Print and shaded views of the part. All mm, measured from the part's lowest x, y and z. A direction names the side the tool comes from. Round coordinates to 2 decimals unless told otherwise and drop trailing zeros. Loops run counter-clockwise (first coordinate to the right, second up) from the corner with the lowest first, then second, coordinate; pieces in that order, holes last. Notation, with made-up numbers: (57, -30) - (89, -30) arc R25 cw to (89, -13) - close; hole circle Ø9 at (0, 12). An arc over 180 degrees is marked (long way). Use one line per item in the form item = value. Start each with the question number.
Q1. Saw through at C-C (z = 3.5). Give the cut face in (x, y) (1 decimal).
Q2. Saw through at B-B (x = 5.5). Give the cut face in (y, z).
Q3. Mould opens along X. For the marked faces 1, 2 and 3 say: released by +X, released by -X, zero draft, split by the parting line, or undercut.
Q4. Pin check, flat tips, straight feed: pin 1 (1 mm diameter, centred on y = 13.5, z = 5.5, fed in from +X); pin 2 (10 mm diameter, centred on x = 10, y = 10.5, fed in from +Z); pin 3 (1 mm diameter, centred on x = 2.5, z = 1.5, fed in from -Y); pin 4 (1.5 mm diameter, centred on x = 13, z = 7, fed in from -Y). Stop position of each tip, or through.
Q5. Saw through at A-A (y = 10). Give the cut face in (x, z).
Q6. 3-axis set-ups, long thin cutter, end or side, ignore diameter. For the marked faces 4 and 5: which of +Z, -Z, +X, -X, +Y, -Y reach the whole face in a straight line?
Q7. Drill centre lines: line 1 (Y direction, x = 10.5, z = 3.5); line 2 (Y direction, x = 4, z = 4) (1 decimal); line 3 (Y direction, x = 7.75, z = 7). Where is each one in solid material? Low to high.
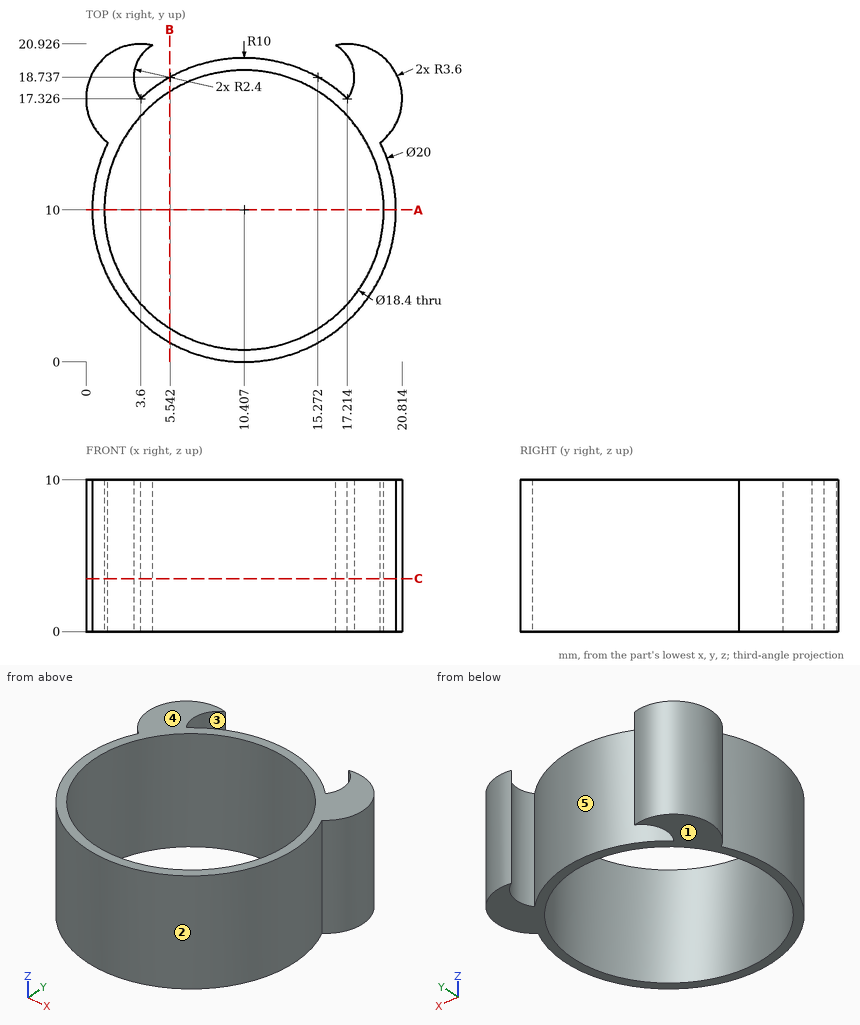
Report:
q1.outline = (1.4, 14.4) arc R10 ccw (long way) to (19.4, 14.4) arc R3.6 ccw to (16.4, 20.8) arc R2.4 cw to (17.2, 17.3) arc R10 ccw to (3.6, 17.3) arc R2.4 cw to (4.4, 20.8) arc R3.6 ccw to start; hole circle Ø18.4 at (10.4, 10)
q2.outline = (1.29, 0) - (2.22, 0) - (2.22, 10) - (1.29, 10) - close; (17.78, 0) - (18.71, 0) - (18.71, 10) - (17.78, 10) - close
q3.face_1 = zero draft
q3.face_2 = split by the parting line
q3.face_3 = undercut
q4.pin_1 = 19.95
q4.pin_2 = through
q4.pin_3 = 3.28
q4.pin_4 = 0.17
q5.outline = (0.41, 0) - (1.21, 0) - (1.21, 10) - (0.41, 10) - close; (19.61, 0) - (20.41, 0) - (20.41, 10) - (19.61, 10) - close
q6.face_4 = +Z, +X, -X, +Y, -Y
q6.face_5 = +Z, -Z
q7.line_1 = 0 to 0.8, 19.2 to 20
q7.line_2 = 2.3 to 3.4, 16.6 to 17.7, 20.6 to 20.9
q7.line_3 = 0.36 to 1.19, 18.81 to 19.64
